from build123d import *

# Parameters (mm, degrees)
SKETCH1_W           = 100
SKETCH1_H           = 380
BOSS_EXTRUDE1_DEPTH = 3
SKETCH1_4_R         = 2.9
SKETCH1_4_R_2       = 4.2
SKETCH1_4_R_3       = 21.25
CUT_EXTRUDE1_DEPTH  = 10


with BuildPart() as part:
    # Sketch1 → Boss-Extrude1 (new body)
    with BuildSketch(Plane.XY):
        with Locations((50, 190)):
            Rectangle(SKETCH1_W, SKETCH1_H)
    extrude(amount=-BOSS_EXTRUDE1_DEPTH)

    # Sketch1<4> → Cut-Extrude1 (cut)
    with BuildSketch(Plane.XY):
        with Locations((24, 100)):
            Circle(SKETCH1_4_R)
        with Locations((76, 100)):
            Circle(SKETCH1_4_R)
        with Locations((24, 46)):
            Circle(SKETCH1_4_R)
        with BuildLine():
            Line((54.75, 58.3), (54.75, 63.689387775))
            ThreePointArc((54.75, 63.689387775), (72.581133525, 76.075464159), (50.916994756, 77.5))
            Line((50.916994756, 77.5), (49.083005244, 77.5))
            ThreePointArc((49.083005244, 77.5), (27.418866475, 76.075464159), (45.25, 63.689387775))
            Line((45.25, 63.689387775), (45.25, 58.3))
            Line((45.25, 58.3), (50, 58.3))
            Line((50, 58.3), (54.75, 58.3))
        make_face()
        with Locations((50, 300.75)):
            Circle(SKETCH1_4_R_2)
        with Locations((50, 258.75)):
            Circle(SKETCH1_4_R_3)
        with Locations((50, 216.75)):
            Circle(SKETCH1_4_R_2)
        with Locations((76, 46)):
            Circle(SKETCH1_4_R)
    extrude(amount=-CUT_EXTRUDE1_DEPTH, mode=Mode.SUBTRACT)


solid = part.part
Read the model definition and answer for the solid it produces. Units are mm, in the model's axes. Round coordinates to 2 decimals unless told otherwise and drop trailing zeros. Loops run counter-clockwise (first coordinate to the right, second up) from the corner with the lowest first, then second, coordinate; pieces in that order, holes last.
Q1. Section D-D on x = 38.5 is taken. Write down the section's boundary in (y, z), and give its area (3 significant figures).
Q2. Section A-A on z = -2.2 is taken. Give the number of separate pieces and of enclosed holes in the cut face, and give its area (3 significant figures).
Q3. Consider probe 1 along Y at (x, z) = (50, -0.8); probe 2 along Y at (x, z) = (24, -1.7); probe 3 along X at (y, z) = (300.75, -1.35). Determine where each line is inside the solid, lowest interval first.
Q4. Determine the mould class of faces 1 (the face through (47.23, 279.82, -1.48)), 2 (the face through (49, 193, 0)) for opening direction Y: released by +Y, released by -Y, zero draft, split by the parting line, or undercut.
Q5. Section B-B on y = 300.75 is taken. Write down the section's boundary in (x, z), and give its area (3 significant figures).
Q6. Section C-C on x = 58.5 is taken. Write down the section's boundary in (y, z), and give its area (3 significant figures).
Output:
1. outline: (0, -3) - (61.5, -3) - (61.5, 0) - (0, 0) - close; (84.5, -3) - (240.88, -3) - (240.88, 0) - (84.5, 0) - close; (276.62, -3) - (380, -3) - (380, 0) - (276.62, 0) - close
1. area: 964 mm2
2. separate pieces: 1
2. enclosed holes: 8
2. area: 35,500 mm2
3. probe 1: y = 0 to 58.3, 77.5 to 212.55, 220.95 to 237.5, 280 to 296.55, 304.95 to 380
3. probe 2: y = 0 to 43.1, 48.9 to 97.1, 102.9 to 380
3. probe 3: x = 0 to 45.8, 54.2 to 100
4. face 1: undercut
4. face 2: zero draft
5. outline: (0, -3) - (45.8, -3) - (45.8, 0) - (0, 0) - close; (54.2, -3) - (100, -3) - (100, 0) - (54.2, 0) - close
5. area: 275 mm2
6. outline: (0, -3) - (61.9, -3) - (61.9, 0) - (0, 0) - close; (84.1, -3) - (239.27, -3) - (239.27, 0) - (84.1, 0) - close; (278.23, -3) - (380, -3) - (380, 0) - (278.23, 0) - close
6. area: 957 mm2
